Geometry: see drawing. Coordinates: mm, zero at the bounding-box minimum. A direction names the side the tool comes from. Give positions to 0.01 mm unless a question says otherwise; leave off trailing zeros. Loops run counter-clockwise (first coordinate to the right, second up) from the corner with the lowest first, then second, coordinate; pieces in that order, holes last. Notation, with made-up numbers: M 20,1.25 L 44,1.25 A25 ccw 44,31.25 Z; hole C 25,-23.5 d5. An arc over 180 degrees is marked long. Put each result on its own line as item: value.
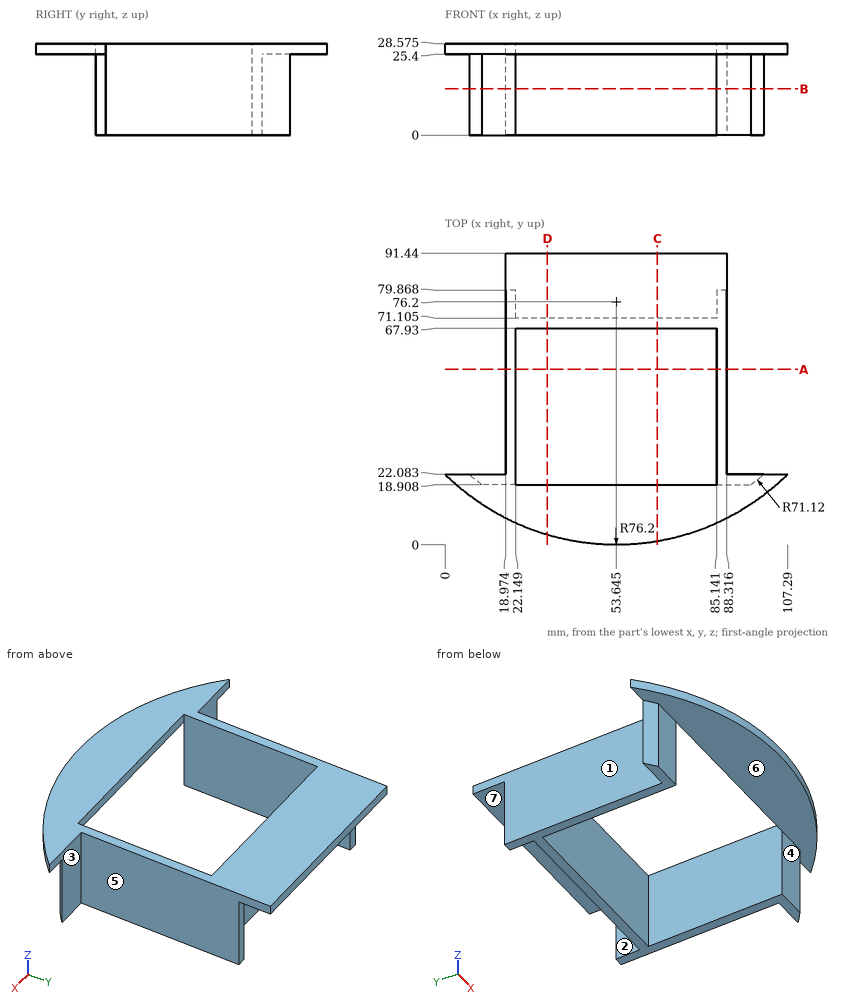
1. Section query C-C (x = 66.5). Output: boundary loops of the cut face in (y, z) (1 decimal), plus the area to 3 significant figures.
Found:
outline: M 1.1,25.4 L 18.9,25.4 L 18.9,28.6 L 1.1,28.6 Z; M 67.9,0 L 71.1,0 L 71.1,25.4 L 91.4,25.4 L 91.4,28.6 L 67.9,28.6 Z
area: 212 mm^2
2. Section query D-D (x = 32). Output: boundary loops of the cut face in (y, z) (1 decimal), plus the area to 3 significant figures.
Found:
outline: M 3.1,25.4 L 18.9,25.4 L 18.9,28.6 L 3.1,28.6 Z; M 67.9,0 L 71.1,0 L 71.1,25.4 L 91.4,25.4 L 91.4,28.6 L 67.9,28.6 Z
area: 205 mm^2
3. Section query A-A (y = 55). Output: boundary loops of the cut face in (x, z) (1 decimal).
Found:
outline: M 19,0 L 22.1,0 L 22.1,28.6 L 19,28.6 Z; M 85.1,0 L 88.3,0 L 88.3,28.6 L 85.1,28.6 Z
4. Section query B-B (z = 14.5). Output: boundary loops of the cut face in (x, y) (1 decimal).
Found:
outline: M 7.5,22.1 A71.1 ccw 11.5,18.9 L 22.1,18.9 L 22.1,67.9 L 85.1,67.9 L 85.1,18.9 L 95.8,18.9 A71.1 ccw 99.8,22.1 L 88.3,22.1 L 88.3,79.9 L 85.1,79.9 L 85.1,71.1 L 22.1,71.1 L 22.1,79.9 L 19,79.9 L 19,22.1 Z
5. Draft query along X for the marked faces 5, 6 and 7. Return one class per face: pulls with the +X half, pulls with the -X half, needs draft (parallel to the pull), parting line crosses it, or undercut.
Found:
face 5: pulls with the +X half
face 6: needs draft
face 7: undercut
6. Material intervals for line 1 (X direction, y = 42, z = 5.25); line 2 (Y direction, x = 69, z = 10.25) (1 decimal); line 3 (Z direction, x = 66, y = 73.5) (1 decimal), sorted ascending. Write a range as from..to.
Found:
line 1: 18.97..22.15, 85.14..88.32
line 2: 67.9..71.1
line 3: 25.4..28.6
7. Contact query for flat-ended pins moving along their axis: P1, Ø6, axis at x = 53.5, y = 81.5, coming from the -Z side; P2, Ø1.5, axis at x = 56.5, z = 12.5, coming from the -Y side; P3, Ø1, axis at x = 87.5, z = 8.5, coming from the +Y side; P4, Ø8, axis at x = 90, y = 55.5, coming from the -Z side. Output: stop coordinate, or through.
Found:
P1: z = 25.4
P2: y = 67.93
P3: y = 79.87
P4: z = 0
8. Access query for the marked faces 1, 2, 3 and 4. Directions: +Z, -Z, +X, -X, +Y, -Y. A direction counts if a zero-diameter tool reaches every point of the face in a straight line with its end or side. Return the directions, or none.
Found:
face 1: +Z, -Z, -X, +Y
face 2: -Z, +Y
face 3: +Z, -Z, +X, +Y
face 4: -Z, +X, -X, -Y
